Could you check a few things on this model? Use its own coordinates, in mm. A direction names the side the tool comes from. Coordinates: 2 decimals unless noted, no trailing zeros. Order: outer loops, then holes, each group sorted by start corner. A loop starts at its lowest first (then second) coordinate and runs counter-clockwise, first axis right, second up.
```python
from build123d import *

# Parameters (mm, degrees)
ESQUISSE1_W             = 199
ESQUISSE1_H             = 48
BOSS_EXTRU_1_DEPTH      = 6
ESQUISSE2_W             = 20
ESQUISSE2_H             = 6
BOSS_EXTRU_2_DEPTH      = 6
ESQUISSE3_W             = 6
ESQUISSE3_H             = 20
BOSS_EXTRU_3_DEPTH      = 6
ESQUISSE4_W             = 78
ESQUISSE4_H             = 5
ENL_V_MAT_EXTRU_1_DEPTH = 213.077815907
ENL_V_MAT_EXTRU_2_DEPTH = 213.077815907
ESQUISSE6_R             = 1.005
ENL_V_MAT_EXTRU_3_DEPTH = 213.077815907
ESQUISSE7_R             = 2
ENL_V_MAT_EXTRU_4_DEPTH = 3
ESQUISSE8_W             = 90
ESQUISSE8_H             = 6
ENL_V_MAT_EXTRU_5_DEPTH = 213.077815907


with BuildPart() as part:
    # Esquisse1 → Boss.-Extru.1 (new body)
    with BuildSketch(Plane.XY):
        with Locations((-99.5, 24)):
            Rectangle(ESQUISSE1_W, ESQUISSE1_H)
    extrude(amount=BOSS_EXTRU_1_DEPTH)

    # Esquisse2 → Boss.-Extru.2 (add)
    with BuildSketch(Plane(origin=(0, 48, 0), x_dir=(1, 0, 0), z_dir=(0, 1, 0))):
        with Locations((-99, -3)):
            Rectangle(ESQUISSE2_W, ESQUISSE2_H)
        with Locations((-159, -3)):
            Rectangle(ESQUISSE2_W, ESQUISSE2_H)
    extrude(amount=BOSS_EXTRU_2_DEPTH)

    # Esquisse3 → Boss.-Extru.3 (add)
    with BuildSketch(Plane.ZY.offset(199)):
        with Locations((3, 24)):
            Rectangle(ESQUISSE3_W, ESQUISSE3_H)
    extrude(amount=BOSS_EXTRU_3_DEPTH)

    # Esquisse4 → Enlèv. mat.-Extru.1 (cut, through all)
    with BuildSketch(Plane.XY.offset(6)):
        with Locations((-39, 2.5)):
            Rectangle(ESQUISSE4_W, ESQUISSE4_H)
    extrude(amount=-ENL_V_MAT_EXTRU_1_DEPTH, mode=Mode.SUBTRACT)

    # Esquisse5 → Enlèv. mat.-Extru.2 (cut, through all)
    with BuildSketch(Plane.XY.offset(6)):
        Polygon((0, 48), (-40, 48), (0, 5), align=None)
    extrude(amount=-ENL_V_MAT_EXTRU_2_DEPTH, mode=Mode.SUBTRACT)

    # Esquisse6 → Enlèv. mat.-Extru.3 (cut, through all)
    with BuildSketch(Plane.XY.offset(6)):
        with Locations((-148.88, 14.5)):
            Circle(ESQUISSE6_R)
        with Locations((-148.88, 30.5)):
            Circle(ESQUISSE6_R)
        with Locations((-132.88, 14.5)):
            Circle(ESQUISSE6_R)
        with Locations((-132.88, 30.5)):
            Circle(ESQUISSE6_R)
        with Locations((-116.88, 14.5)):
            Circle(ESQUISSE6_R)
        with Locations((-116.88, 30.5)):
            Circle(ESQUISSE6_R)
        with Locations((-100.88, 14.5)):
            Circle(ESQUISSE6_R)
        with Locations((-100.88, 30.5)):
            Circle(ESQUISSE6_R)
        with Locations((-84.88, 14.5)):
            Circle(ESQUISSE6_R)
        with Locations((-84.88, 30.5)):
            Circle(ESQUISSE6_R)
        with Locations((-68.88, 14.5)):
            Circle(ESQUISSE6_R)
        with Locations((-68.88, 30.5)):
            Circle(ESQUISSE6_R)
        with Locations((-52.88, 14.5)):
            Circle(ESQUISSE6_R)
        with Locations((-52.88, 30.5)):
            Circle(ESQUISSE6_R)
        with Locations((-164.88, 14.5)):
            Circle(ESQUISSE6_R)
        with Locations((-164.88, 30.5)):
            Circle(ESQUISSE6_R)
        with Locations((-180.88, 14.5)):
            Circle(ESQUISSE6_R)
        with Locations((-180.88, 30.5)):
            Circle(ESQUISSE6_R)
    extrude(amount=-ENL_V_MAT_EXTRU_3_DEPTH, mode=Mode.SUBTRACT)

    # Esquisse7 → Enlèv. mat.-Extru.4 (cut)
    with BuildSketch(Plane.XY.offset(6)):
        with Locations((-52.88, 14.5)):
            Circle(ESQUISSE7_R)
        with Locations((-52.88, 30.5)):
            Circle(ESQUISSE7_R)
        with Locations((-68.88, 14.5)):
            Circle(ESQUISSE7_R)
        with Locations((-68.88, 30.5)):
            Circle(ESQUISSE7_R)
        with Locations((-84.88, 14.5)):
            Circle(ESQUISSE7_R)
        with Locations((-84.88, 30.5)):
            Circle(ESQUISSE7_R)
        with Locations((-100.88, 14.5)):
            Circle(ESQUISSE7_R)
        with Locations((-100.88, 30.5)):
            Circle(ESQUISSE7_R)
        with Locations((-116.88, 14.5)):
            Circle(ESQUISSE7_R)
        with Locations((-116.88, 30.5)):
            Circle(ESQUISSE7_R)
        with Locations((-132.88, 14.5)):
            Circle(ESQUISSE7_R)
        with Locations((-132.88, 30.5)):
            Circle(ESQUISSE7_R)
        with Locations((-148.88, 14.5)):
            Circle(ESQUISSE7_R)
        with Locations((-148.88, 30.5)):
            Circle(ESQUISSE7_R)
        with Locations((-164.88, 14.5)):
            Circle(ESQUISSE7_R)
        with Locations((-164.88, 30.5)):
            Circle(ESQUISSE7_R)
        with Locations((-180.88, 14.5)):
            Circle(ESQUISSE7_R)
        with Locations((-180.88, 30.5)):
            Circle(ESQUISSE7_R)
    extrude(amount=-ENL_V_MAT_EXTRU_4_DEPTH, mode=Mode.SUBTRACT)

    # Esquisse8 → Enlèv. mat.-Extru.5 (cut, through all)
    with BuildSketch(Plane(origin=(0, 0, 0), x_dir=(-1, 0, 0), z_dir=(0, 0, -1))):
        with Locations((154, 3)):
            Rectangle(ESQUISSE8_W, ESQUISSE8_H)
    extrude(amount=-ENL_V_MAT_EXTRU_5_DEPTH, mode=Mode.SUBTRACT)


solid = part.part
```
Item 1: Thinking about a two-plate mould opening in X: for faces 5 (the face through (-109, 3, 3)), 6 (the face through (-159, 54, 3)), 7 (the face through (-166, 14, 3)), 8 (the face through (-129, 48, 3)), which applies, +X half, -X half, draft (parallel to the pull), parting line (faces both ways), or undercut?
Item 2: I need wall thicknesses on line 1 (Y direction, x = -52.88, z = 1.7) (3 decimals); line 2 (Y direction, x = -180.88, z = 3.75); line 3 (Y direction, x = -46, z = 2.75). Which ranges of each line are inside material? Lowest first, please.
Item 3: For pin 1 Ø3 at (x, y) = (-132.88, 30.5) entering from +Z; pin 2 Ø1.2 at (x, y) = (-164.88, 14.5) entering from -Z; pin 3 Ø1 at (y, z) = (45, 2) entering from +X; pin 4 Ø1 at (x, z) = (-135.5, 4.5) entering from -Y, each with a flat end and sliding along its axis, tell me the tip position at first contact or that it passes through.
Item 4: Suppose I cut it at A-A (z = 1.15). Count the separate pieces of the cut face and the enclosed holes in it, and give its area (3 significant figures).
Item 5: Suppose I cut it at B-B (y = 21). List the corners of the cut face in (x, z) for me.
Item 6: Which directions (+Z, -Z, +X, -X, +Y, -Y) give clear straight access to the entire face, cutting with the end or side of a thin tool? Please do faces 1 (the face through (-202, 34, 3)), 2 (the face through (-109, 51, 3)), 3 (the face through (-40, 5, 3)), 4 (the face through (-182, 14, 3)).
Item 7: Suppose I cut it at C-C (x = -33). List the corners of the cut face in (y, z) for me (3 decimals).
Geometry results:
1. face 5: -X half
1. face 6: draft
1. face 7: undercut
1. face 8: undercut
2. line 1: y = 5 to 13.495, 15.505 to 29.495, 31.505 to 48
2. line 2: y = 6 to 12.5, 16.5 to 28.5, 32.5 to 48
2. line 3: y = 5 to 48
3. pin 1: stops at z = 3
3. pin 2: passes through
3. pin 3: stops at x = -36.74
3. pin 4: stops at y = 6
4. separate pieces: 1
4. enclosed holes: 18
4. area: 8,060 mm2
5. outline: (-205, 0) - (-14.88, 0) - (-14.88, 6) - (-205, 6) - close
6. face 1: +Z, -Z, -X, +Y
6. face 2: +Z, -Z, +Y
6. face 3: +Z, -Z, +X, -Y
6. face 4: +Z
7. outline: (5, 0) - (40.475, 0) - (40.475, 6) - (5, 6) - close
